For this review, use the dimensioned drawing (mm, ordinates from the lowest corner) and the shaded views. A direction names the side the tool comes from. Coordinates: 2 decimals unless noted, no trailing zeros. Write each loop counter-clockwise with the first axis right and the second up, starting at its lowest first coordinate (ties: lowest second). Pieces come first, ordered by that corner, then holes.
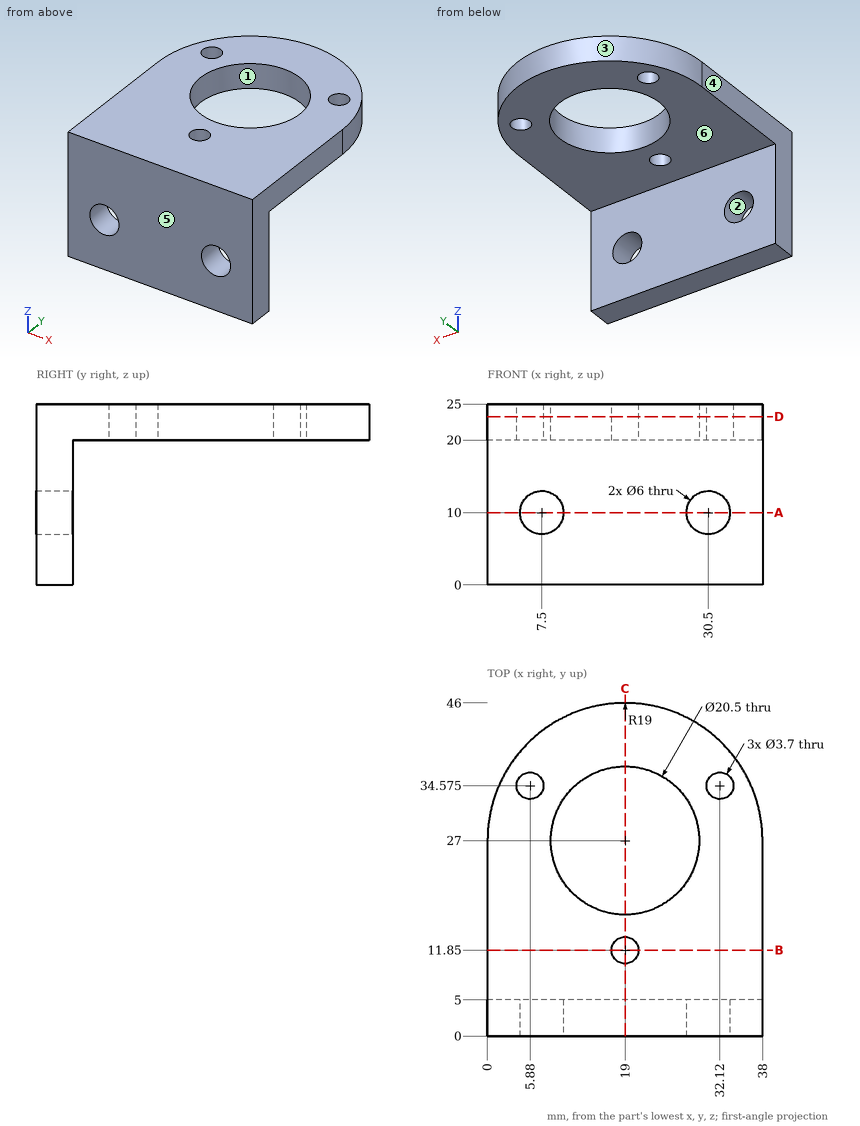
(1) Consider section A-A (z = 10). Give the boundary of the cut face in (x, y).
(2) Wall thickness on line 1 (Y direction, x = 19, z = 23.3); line 2 (X direction, y = 3.05, z = 10); line 3 (Z direction, x = 30.5, y = 3.9): over which ranges is each line inside the solid? List them lowest first.
(3) Consider section B-B (y = 11.85). Give the boundary of the cut face in (x, z).
(4) Consider section D-D (z = 23.25). State how many separate pieces and enclosed holes the cut face has, plus the area to 3 significant figures.
(5) Insertion check: pin 1 Ø19 at (x, y) = (21, 35.5) entering from -Z; pin 2 Ø4.5 at (x, y) = (32.12, 34.58) entering from +Z; pin 3 Ø7 at (x, z) = (30.5, 10) entering from +Y. Each pin has a flat end and moves straight along its axis. Give the tip position at first contact, or say it passes through.
(6) Mouldability with a two-part tool opening along X and no side actions: class the marked faces 1, 2, 3 and 4 as +X half, -X half, draft (parallel to the pull), parting line (faces both ways), or undercut.
(7) For the marked faces 5 and 6, list the 3-axis set-ups (+Z, -Z, +X, -X, +Y, -Y) from which the entire face can be reached by the end or side of a thin tool; tool diameter is ignored.
(8) Consider section C-C (x = 19). Give the boundary of the cut face in (y, z).
Results:
1. outline: (0, 0) - (4.5, 0) - (4.5, 5) - (0, 5) - close; (10.5, 0) - (27.5, 0) - (27.5, 5) - (10.5, 5) - close; (33.5, 0) - (38, 0) - (38, 5) - (33.5, 5) - close
2. line 1: y = 0 to 10, 13.7 to 16.75, 37.25 to 46
2. line 2: x = 0 to 4.5, 10.5 to 27.5, 33.5 to 38
2. line 3: z = 0 to 7, 13 to 25
3. outline: (0, 20) - (17.15, 20) - (17.15, 25) - (0, 25) - close; (20.85, 20) - (38, 20) - (38, 25) - (20.85, 25) - close
4. separate pieces: 1
4. enclosed holes: 4
4. area: 1,230 mm2
5. pin 1: stops at z = 20
5. pin 2: stops at z = 25
5. pin 3: stops at y = 5
6. face 1: undercut
6. face 2: undercut
6. face 3: parting line
6. face 4: -X half
7. face 5: +Z, -Z, +X, -X, -Y
7. face 6: -Z, +X, -X, +Y
8. outline: (0, 0) - (5, 0) - (5, 20) - (10, 20) - (10, 25) - (0, 25) - close; (13.7, 20) - (16.75, 20) - (16.75, 25) - (13.7, 25) - close; (37.25, 20) - (46, 20) - (46, 25) - (37.25, 25) - close
